Here's how the part is built. I have some questions about the finished solid (model axes, mm). Face numbers are marked on the shaded views. A direction names the side the tool comes from. Give positions to 0.01 mm unless a question says otherwise; leave off trailing zeros. Write each loop counter-clockwise with the first axis right and the second up, starting at its lowest first coordinate (ties: lowest second). Pieces come first, ordered by that corner, then holes. Notation, with made-up numbers: (-38, 4) -> (-11, 4) arc R11 ccw to (-11, 12) -> close; hole circle Ø11 at (65.5, 67). An arc over 180 degrees is marked (long way). Put each result on its own line as item: value. Start each with the question number.
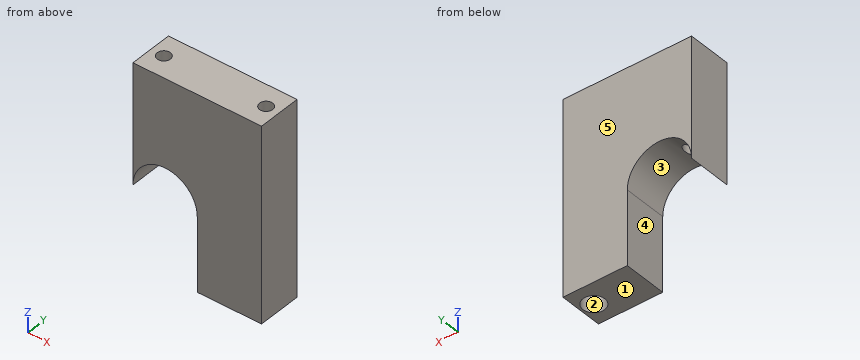
from build123d import *

# Parameters (mm, degrees)
BOSS_EXTRUDE1_DEPTH            = 15
SKETCH11_W                     = 2.25
SKETCH11_H                     = 12.7
M4_CLEARANCE_HOLE5_AT_2_COUNT  = 2
M4_CLEARANCE_HOLE5_AT_2_PITCH  = 35
SKETCH13_W                     = 3.75
SKETCH13_H                     = 53.7
F_6_0MM_DOWEL_HOLE1_AT_2_COUNT = 2
F_6_0MM_DOWEL_HOLE1_AT_2_PITCH = 35


with BuildPart() as part:
    # Sketch1 → Boss-Extrude1 (new body)
    with BuildSketch(Plane(origin=(0, 0, 0), x_dir=(1, 0, 0), z_dir=(0, 1, 0))):
        with BuildLine():
            Line((0, 0), (0, 41))
            ThreePointArc((0, 41), (11, 30), (22, 41))
            Line((22, 41), (22, 66.4))
            Line((22, 66.4), (44, 66.4))
            Line((44, 66.4), (44, 41))
            Line((44, 41), (44, 0))
            Line((44, 0), (0, 0))
        make_face()
    extrude(amount=BOSS_EXTRUDE1_DEPTH)

    # Sketch11 → M4 Clearance Hole5 (revolve, cut)
    with BuildSketch(Plane(origin=(39.5, 7.5, -12.7), x_dir=(0, 1, 0), z_dir=(1, 0, 0))):
        with Locations((1.125, 6.35)):
            Rectangle(SKETCH11_W, SKETCH11_H)
    m4_clearance_hole5 = revolve(axis=Axis((39.5, 7.5, -19.05), (0, 0, 1)), mode=Mode.SUBTRACT)

    # M4 Clearance Hole5 at 2: M4 Clearance Hole5 ×2
    with Locations(*[(-i * M4_CLEARANCE_HOLE5_AT_2_PITCH, 0, 0) for i in range(1, M4_CLEARANCE_HOLE5_AT_2_COUNT)]):
        add(m4_clearance_hole5, mode=Mode.SUBTRACT)

    # Sketch13 → Ø6.0mm Dowel Hole1 (revolve, cut)
    with BuildSketch(Plane(origin=(39.5, 7.5, -12.7), x_dir=(0, -1, 0), z_dir=(1, 0, 0))):
        with Locations((1.875, 26.85)):
            Rectangle(SKETCH13_W, SKETCH13_H)
    f_6_0mm_dowel_hole1 = revolve(axis=Axis((39.5, 7.5, -6.35), (0, 0, -1)), mode=Mode.SUBTRACT)

    # Ø6.0mm Dowel Hole1 at 2: Ø6.0mm Dowel Hole1 ×2
    with Locations(*[(-i * F_6_0MM_DOWEL_HOLE1_AT_2_PITCH, 0, 0) for i in range(1, F_6_0MM_DOWEL_HOLE1_AT_2_COUNT)]):
        add(f_6_0mm_dowel_hole1, mode=Mode.SUBTRACT)


solid = part.part
1) Which directions (+Z, -Z, +X, -X, +Y, -Y) give clear straight access to the entire face, cutting with the end or side of a thin tool? Please do the marked faces 1 and 2.
2) I want a section at A-A, the plane x = 39.5. Write out the boundary of the cut face in (y, z), and give its area (3 significant figures).
3) Thinking about a two-plate mould opening in X: for the marked faces 3, 4 and 5, which applies, released by +X, released by -X, zero draft, split by the parting line, or undercut?
4) I want a section at D-D, the plane x = 4.5. Write out the boundary of the cut face in (y, z), and give its area (3 significant figures).
5) I want a section at B-B, the plane z = -15. Write out the boundary of the cut face in (x, y), and give its area (3 significant figures).
6) I want a section at C-C, the plane y = 6.25. Write out the boundary of the cut face in (x, z), and give its area (3 significant figures).
7) I'm going to push flat-ended pins straight in: pin 1 Ø4.5 at (y, z) = (4.5, -50) entering from -X; pin 2 Ø6 at (x, y) = (14.5, 4.5) entering from -Z; pin 3 Ø2.5 at (x, y) = (4.5, 7.5) entering from +Z. Where does each tip first touch, or does it pass through?
8) I need wall thicknesses on probe 1 along X at (y, z) = (7.5, -25); probe 2 along X at (y, z) = (7.5, -6.25); probe 3 along Y at (x, z) = (4.5, -4.75). Which ranges of each line are inside material? Lowest first, please.
Established:
1. face 1: -Z, +X, -X, +Y, -Y
1. face 2: -Z
2. outline: (0, -66.4) -> (3.75, -66.4) -> (3.75, -12.7) -> (5.25, -12.7) -> (5.25, 0) -> (0, 0) -> close; (9.75, -12.7) -> (11.25, -12.7) -> (11.25, -66.4) -> (15, -66.4) -> (15, 0) -> (9.75, 0) -> close
2. area: 536 mm2
3. face 3: undercut
3. face 4: released by -X
3. face 5: zero draft
4. outline: (0, -32.13) -> (3.75, -32.13) -> (3.75, -12.7) -> (5.25, -12.7) -> (5.25, 0) -> (0, 0) -> close; (9.75, -12.7) -> (11.25, -12.7) -> (11.25, -32.13) -> (15, -32.13) -> (15, 0) -> (9.75, 0) -> close
4. area: 279 mm2
5. outline: (0, 0) -> (44, 0) -> (44, 15) -> (0, 15) -> close; hole circle Ø7.5 at (4.5, 7.5); hole circle Ø7.5 at (39.5, 7.5)
5. area: 572 mm2
6. outline: (0, -41) arc R11 cw to (0.96, -36.5) -> (0.96, -12.7) -> (2.63, -12.7) -> (2.63, 0) -> (0, 0) -> close; (6.37, -12.7) -> (8.04, -12.7) -> (8.04, -30.41) arc R11 cw to (22, -41) -> (22, -66.4) -> (35.96, -66.4) -> (35.96, -12.7) -> (37.63, -12.7) -> (37.63, 0) -> (6.37, 0) -> close; (41.37, -12.7) -> (43.04, -12.7) -> (43.04, -66.4) -> (44, -66.4) -> (44, 0) -> (41.37, 0) -> close
6. area: 1,560 mm2
7. pin 1: stops at x = 22
7. pin 2: stops at z = -32.13
7. pin 3: passes through
8. probe 1: x = 0 to 0.75, 8.25 to 35.75, 43.25 to 44
8. probe 2: x = 0 to 2.25, 6.75 to 37.25, 41.75 to 44
8. probe 3: y = 0 to 5.25, 9.75 to 15
